Geometry: final body of the model. Coordinates: model frame, mm. Face numbers are marked on the shaded views. A direction names the side the tool comes from. Round coordinates to 2 decimals unless told otherwise and drop trailing zeros. Write each loop counter-clockwise with the first axis right and the second up, starting at its lowest first coordinate (ties: lowest second). Pieces come first, ordered by that corner, then holes. Notation, with made-up numbers: M 57.25,71.25 L 81.25,71.25 A6 ccw 81.25,76.25 Z; hole C -35,35.5 d6. An arc over 180 degrees is marked long. Put each result on its own line as item: value. Start each with the question number.
```python
from build123d import *

# Parameters (mm, degrees)
F0_W     = 3
F0_H     = 30
F0_H_2   = 32
F1_DEPTH = 14
F3_D     = 2
F3_DEPTH = 12
F3_TIP   = 0.600860619
F4_W     = 4.5
F4_H     = 4.5
F5_DEPTH = 2
F7_D     = 4.2
F8_SIZE  = 9.99999
F9_SIZE  = 1.99999


# Not quite as in the source:
# - a fillet or chamfer is up to 0.001 mm smaller than in the source, because OpenCascade refuses the exact size


with BuildPart() as f1:
    # F0 (on Top) → F1 (new body)
    with BuildSketch(Plane.XY):
        with Locations((-31.0656790137, 37.4089360237)):
            Rectangle(F0_W, F0_H)
        Polygon((-29.5656790137, 22.4089360237), (-32.5656790137, 22.4089360237), (-42.5656790137, 22.4089360237), (-42.5656790137, 19.4089360237), (-39.5656790137, 19.4089360237), (-29.5656790137, 19.4089360237), align=None)
        with Locations((-41.0656790137, 3.4089360237)):
            Rectangle(F0_W, F0_H_2)
    extrude(amount=F1_DEPTH)

    # F3
    with Locations(Plane.YZ.offset(-29.5656790137)):
        with Locations((47.4089360237, 11), (47.4089360237, 3)):
            Hole(F3_D / 2, depth=F3_DEPTH)
            with Locations((0, 0, -(F3_DEPTH + F3_TIP / 2))):  # 118° drill point
                Cone(0, F3_D / 2, F3_TIP, mode=Mode.SUBTRACT)

    # F4 (on face) → F5 (join)
    with BuildSketch(Plane(origin=(-42.5656790137, 0, 0), x_dir=(0, -1, 0), z_dir=(-1, 0, 0))):
        with Locations((-5.1589360237, 7)):
            Rectangle(F4_W, F4_H)
        with Locations((10.3410639763, 7)):
            Rectangle(F4_W, F4_H)
    extrude(amount=F5_DEPTH)

    # F7 (through all)
    with Locations(Plane.YZ.offset(-39.5656790137)):
        with Locations((-2.5910639763, 7)):
            Hole(F7_D / 2)

    # F8 (size 10 in the source; OpenCascade refuses exactly that, so slightly less here)
    f8_edges = [f1.edges().sort_by_distance(p)[0] for p in [
        (-39.565679, 19.408936, 7),
    ]]
    chamfer(f8_edges, length=F8_SIZE)

    # F9 (size 2 in the source; OpenCascade refuses exactly that, so slightly less here)
    f9_edges = [f1.edges().sort_by_distance(p)[0] for p in [
        (-44.565679, 5.158936, 4.75),
        (-44.565679, -10.341064, 4.75),
        (-44.565679, -10.341064, 9.25),
        (-44.565679, 5.158936, 9.25),
    ]]
    chamfer(f9_edges, length=F9_SIZE)


solid = f1.part
```
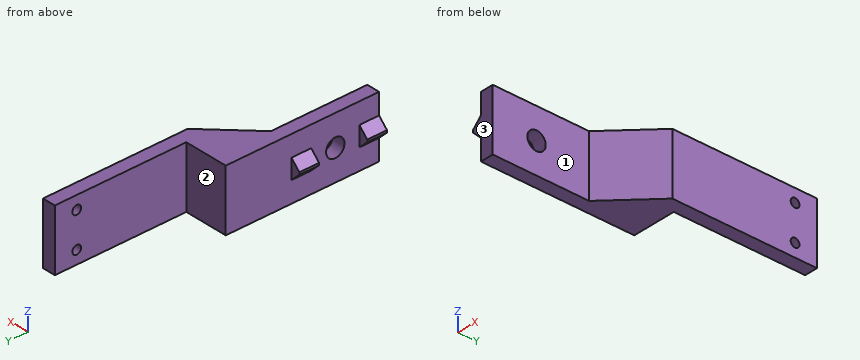
1) Access query for the marked faces 1, 2 and 3. Directions: +Z, -Z, +X, -X, +Y, -Y. A direction counts if a zero-diameter tool reaches every point of the face in a straight line with its end or side. Return the directions, or none.
2) First-contact query: pin 1 (1 mm diameter, centred on x = -44, z = 7, fed in from +Y); pin 2 (4 mm diameter, centred on y = 22, z = 6.5, fed in from -X); pin 3 (5 mm diameter, centred on x = -37, z = 10, fed in from -Y). Flat tips, straight axial feed; report the tip coordinate or a pass-through.
3) Ray query, probe 1 along X at (y, z) = (24.5, 4.25); probe 2 along X at (y, z) = (19.5, 3.5); probe 3 along Y at (x, z) = (-30, 2.75). Return the intervals inside material, ascending.
4) Section B-B, the plane y = -4. Output: boundary loops of the cut face in (x, z).
5) Section C-C, the plane x = -31.25. Output: boundary loops of the cut face in (y, z), and give its area (3 significant figures).
Solved:
1. face 1: +Z, -Z, +X, -Y
1. face 2: +Z, -Z, -X, +Y
1. face 3: +Z, -Z, +X, -X, -Y
2. pin 1: stops at y = 7.41
2. pin 2: stops at x = -42.57
2. pin 3: stops at y = 9.47
3. probe 1: x = -32.57 to -29.57
3. probe 2: x = -42.57 to -29.57
3. probe 3: y = 18.97 to 46.44, 48.38 to 52.41
4. outline: M -42.57,0 L -39.57,0 L -39.57,5.44 L -42.57,5.44 Z; M -42.57,8.56 L -39.57,8.56 L -39.57,14 L -42.57,14 Z
5. outline: M 17.72,0 L 52.41,0 L 52.41,14 L 17.72,14 Z; hole C 47.41,3 d2; hole C 47.41,11 d2
5. area: 479 mm2
